from build123d import *

# Parameters (mm, degrees)
BOSS_EXTRUDE1_DEPTH   = 12
BOSS_EXTRUDE1_2_DEPTH = 12
SKETCH1_W             = 50
SKETCH1_H             = 50
BOSS_EXTRUDE1_3_DEPTH = 12
SKETCH2_W             = 4
SKETCH2_H             = 12.279350853
BOSS_EXTRUDE2_DEPTH   = 3
SKETCH3_W             = 4
SKETCH3_H             = 12.244216487
SKETCH3_H_2           = 12.279350853
BOSS_EXTRUDE3_DEPTH   = 3
SKETCH4_W             = 13.297909738
SKETCH4_H             = 8.9
SKETCH4_R             = 2.5
BOSS_EXTRUDE4_DEPTH   = 1.5


with BuildPart() as part:
    # Sketch1 → Boss-Extrude1 (new body)
    with BuildSketch(Plane.XY):
        with BuildLine():
            Line((-19, 32.908965344), (-20, 34.641016151))
            ThreePointArc((-20, 34.641016151), (0, 40), (20, 34.641016151))
            Line((20, 34.641016151), (19, 32.908965344))
            ThreePointArc((19, 32.908965344), (0, 38), (-19, 32.908965344))
        make_face()
    extrude(amount=BOSS_EXTRUDE1_DEPTH)



with BuildPart() as body_2:
    # Sketch1 → Boss-Extrude1 2 (new body)
    with BuildSketch(Plane.XY):
        with BuildLine():
            Line((19, -32.908965344), (20, -34.641016151))
            ThreePointArc((20, -34.641016151), (0, -40), (-20, -34.641016151))
            Line((-20, -34.641016151), (-19, -32.908965344))
            ThreePointArc((-19, -32.908965344), (0, -38), (19, -32.908965344))
        make_face()
    extrude(amount=BOSS_EXTRUDE1_2_DEPTH)


with BuildPart() as body_3:
    # Sketch1 → Boss-Extrude1 3 (new body)
    with BuildSketch(Plane.XY):
        with BuildLine():
            Line((-30.397368307, 26), (-26, 26))
            Line((-26, 26), (23.958297101, 26))
            Line((23.958297101, 26), (30.397368307, 26))
            ThreePointArc((30.397368307, 26), (40, 0), (30.397368307, -26))
            Line((30.397368307, -26), (23.958297101, -26))
            Line((23.958297101, -26), (-26, -26))
            Line((-26, -26), (-30.397368307, -26))
            ThreePointArc((-30.397368307, -26), (-40, 0), (-30.397368307, 26))
        make_face()
        Rectangle(SKETCH1_W, SKETCH1_H, mode=Mode.SUBTRACT)
    extrude(amount=BOSS_EXTRUDE1_3_DEPTH)


with BuildPart() as part_1:
    add(part.part)

    add(body_2.part)  # Boss-Extrude2 merges body 2

    add(body_3.part)  # Boss-Extrude2 merges body 3
    # Sketch2 → Boss-Extrude2 (add)
    with BuildSketch(Plane.XY.offset(12)):
        with Locations((-9.365459931, 31.139675427)):
            Rectangle(SKETCH2_W, SKETCH2_H)
        with Locations((9.365459931, 31.139675427)):
            Rectangle(SKETCH2_W, SKETCH2_H)
        with Locations((9.365459931, -31.139675427)):
            Rectangle(SKETCH2_W, SKETCH2_H)
        with Locations((-9.365459931, -31.139675427)):
            Rectangle(SKETCH2_W, SKETCH2_H)
    extrude(amount=-BOSS_EXTRUDE2_DEPTH)

    # Sketch3 → Boss-Extrude3 (add)
    with BuildSketch(Plane(origin=(0, 0, 0), x_dir=(-1, 0, 0), z_dir=(0, 0, -1))):
        with Locations((-9.365459931, 31.122108244)):
            Rectangle(SKETCH3_W, SKETCH3_H)
        with Locations((9.365459931, 31.139675427)):
            Rectangle(SKETCH3_W, SKETCH3_H_2)
        with Locations((-9.365459931, -31.139675427)):
            Rectangle(SKETCH3_W, SKETCH3_H_2)
        with Locations((9.365459931, -31.139675427)):
            Rectangle(SKETCH3_W, SKETCH3_H_2)
    extrude(amount=-BOSS_EXTRUDE3_DEPTH)

    # Sketch4 → Boss-Extrude4 (add)
    # profile 1 of 4: a face of its own
    with BuildSketch(Plane.XY.offset(12)):
        with Locations((-23.748413438, -21.55)):
            Rectangle(SKETCH4_W, SKETCH4_H)
        with Locations((-21, -21)):
            Circle(SKETCH4_R, mode=Mode.SUBTRACT)
    # profile 2 of 4: a face of its own
    with BuildSketch(Plane.XY.offset(12)):
        with Locations((23.748413438, -21.55)):
            Rectangle(SKETCH4_W, SKETCH4_H)
        with Locations(Location((21, -21, 0), (0, 0, 180))):
            Circle(SKETCH4_R, mode=Mode.SUBTRACT)
    # profile 3 of 4: a face of its own
    with BuildSketch(Plane.XY.offset(12)):
        with Locations((23.748413438, 21.55)):
            Rectangle(SKETCH4_W, SKETCH4_H)
        with Locations((21, 21)):
            Circle(SKETCH4_R, mode=Mode.SUBTRACT)
    # profile 4 of 4: a face of its own
    with BuildSketch(Plane.XY.offset(12)):
        with Locations((-23.748413438, 21.55)):
            Rectangle(SKETCH4_W, SKETCH4_H)
        with Locations(Location((-21, 21, 0), (0, 0, 180))):
            Circle(SKETCH4_R, mode=Mode.SUBTRACT)
    extrude(amount=-BOSS_EXTRUDE4_DEPTH)


solid = part_1.part
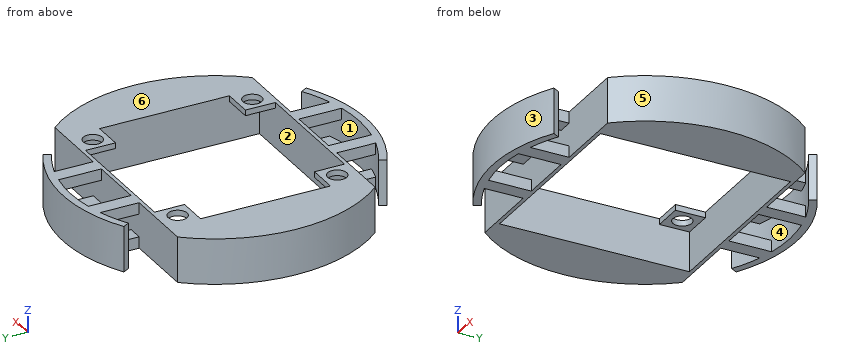
Design review of the part built by this model. Coordinates are the model's own, in mm. Face numbers are marked on the shaded views. A direction names the side the tool comes from. Coordinates: 2 decimals unless noted, no trailing zeros. Loops run counter-clockwise (first coordinate to the right, second up) from the corner with the lowest first, then second, coordinate; pieces in that order, holes last. Notation, with made-up numbers: (46.25, 32.5) - (85.25, 32.5) arc R11 cw to (85.25, 40.5) - close; hole circle Ø11 at (-14.75, 78.25). An arc over 180 degrees is marked (long way). Use CSV: the item, a comma, the result in double quotes. Start each with the question number.
1. Clearance check with flat-ended pins moving along their axes: pin 1 (1.2 mm diameter, centred on x = 20, z = 11, fed in from +Y); pin 2 (0.9 mm diameter, centred on y = -29, z = 10.5, fed in from -X); pin 3 (1.6 mm diameter, centred on y = 21.5, z = 11.5, fed in from +X). State where each tip first meets the part, or that it passes through.
2. Add section B-B on x = -21. Give the boundary of the cut face in (y, z), plus the area to 3 significant figures.
3. Mouldability with a two-part tool opening along Z and no side actions: class the marked faces 4, 5 and 6 as released by +Z, released by -Z, zero draft, split by the parting line, or undercut.
4. Add section D-D on x = -9. Give the boundary of the cut face in (y, z), plus the area to 3 significant figures.
5. Add section C-C on y = 28. Give the boundary of the cut face in (x, z), plus the area to 3 significant figures.
6. Add section A-A on z = 4.5. Give the boundary of the cut face in (x, y), plus the area to 3 significant figures.
7. To check wall thickness, follow probe 1 along Y at (x, z) = (21, 11.1); probe 2 along Y at (x, z) = (15, 6.5); probe 3 along X at (y, z) = (-18.5, 1.75). State the ranges of each line that lie inside material, in increasing order.
8. For the marked faces 1, 2 and 3, list the 3-axis set-ups (+Z, -Z, +X, -X, +Y, -Y) from which the entire face can be reached by the end or side of a thin tool; tool diameter is ignored.
Resolved:
1,pin 1,"y = 34.98"
1,pin 2,"x = -11.37"
1,pin 3,"x = 34.23"
2,outline,"(-26, 0) - (-25, 0) - (-25, 10.5) - (-23.5, 10.5) - (-23.5, 12) - (-26, 12) - close; (-18.5, 10.5) - (-17.1, 10.5) - (-17.1, 12) - (-18.5, 12) - close; (17.1, 10.5) - (18.5, 10.5) - (18.5, 12) - (17.1, 12) - close; (23.5, 10.5) - (25, 10.5) - (25, 0) - (26, 0) - (26, 12) - (23.5, 12) - close"
2,area,"32.7 mm2"
3,face 4,"undercut"
3,face 5,"zero draft"
3,face 6,"released by +Z"
4,outline,"(-38.97, 0) - (-25, 0) - (-25, 12) - (-38.97, 12) - close; (25, 0) - (38.97, 0) - (38.97, 12) - (25, 12) - close; hole (-36.92, 3) - (-26, 3) - (-26, 9) - (-36.92, 9) - close; hole (26, 3) - (36.92, 3) - (36.92, 9) - (26, 9) - close"
4,area,"204 mm2"
5,outline,"(-11.37, 0) - (-7.37, 0) - (-7.37, 3) - (-11.37, 3) - close; (-11.37, 9) - (-7.37, 9) - (-7.37, 12) - (-11.37, 12) - close; (7.37, 0) - (11.37, 0) - (11.37, 3) - (7.37, 3) - close; (7.37, 9) - (11.37, 9) - (11.37, 12) - (7.37, 12) - close"
5,area,"48.0 mm2"
6,outline,"(-30.4, -26) - (30.4, -26) arc R40 ccw to (30.4, 26) - (-30.4, 26) arc R40 ccw to start; (-20, -34.64) arc R40 ccw to (20, -34.64) - (19, -32.91) arc R38 cw to (-19, -32.91) - close; (-20, 34.64) - (-19, 32.91) arc R38 cw to (19, 32.91) - (20, 34.64) arc R40 ccw to start; hole (-25, -25) - (25, -25) - (25, 25) - (-25, 25) - close"
6,area,"1,510 mm2"
7,probe 1,"-26 to -23.5, -18.5 to -17.1, 17.1 to 18.5, 23.5 to 26"
7,probe 2,"-37.08 to -34.91, -26 to -25, 25 to 26, 34.91 to 37.08"
7,probe 3,"-35.46 to -25, 25 to 35.46"
8,face 1,"none"
8,face 2,"-Z"
8,face 3,"+Z, -Z, -Y"
